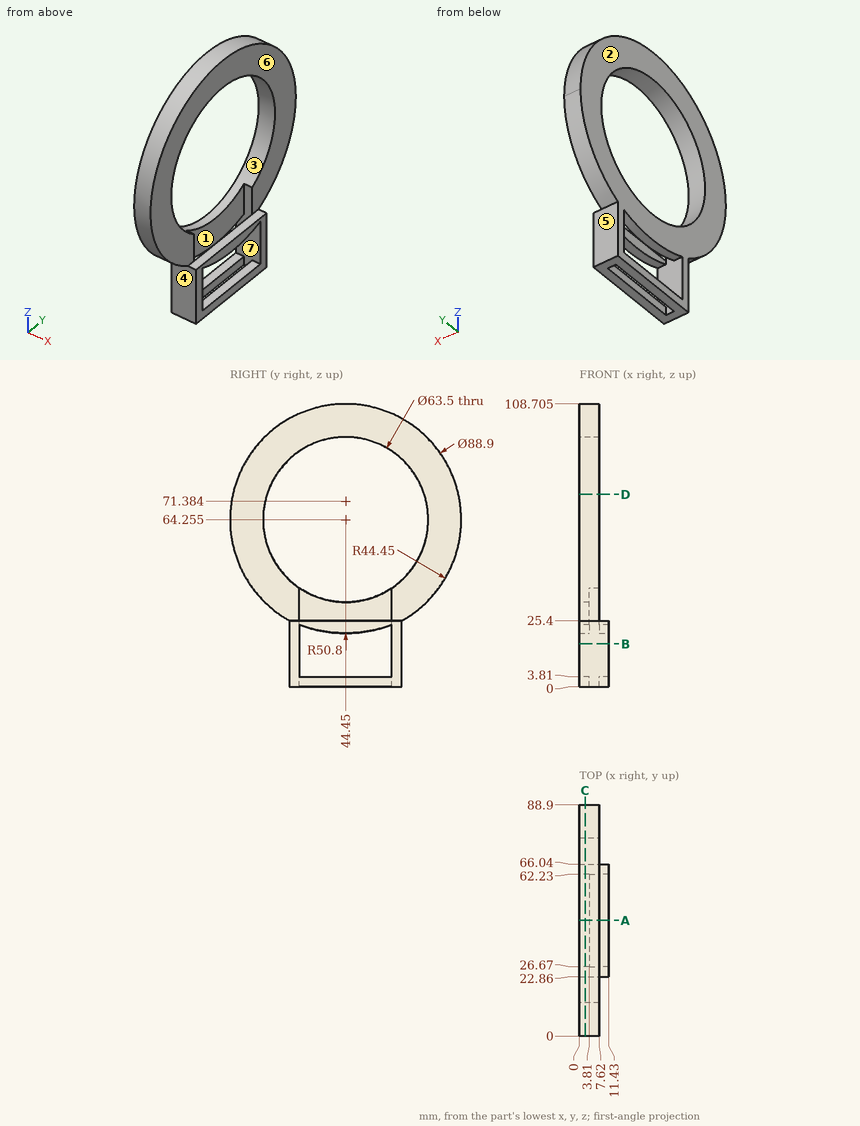
The figure shows three views and two pictorial views of one solid part (mm, origin at its lowest corner). Answer the questions. A direction names the side the tool comes from. Round coordinates to 2 decimals unless told otherwise and drop trailing zeros. Loops run counter-clockwise (first coordinate to the right, second up) from the corner with the lowest first, then second, coordinate; pieces in that order, holes last. Notation, with made-up numbers: M 20.5,53.25 L 52.5,53.25 A21 ccw 52.5,84.25 Z; hole C 8.5,-30 d5. An arc over 180 degrees is marked long. Use CSV: the item, a comma, the result in double quotes.
Q1. Section C-C, the plane x = 2.25 is taken. State how many separate pieces and enclosed holes the cut face has, then the cut area to 3 significant figures.
Determined:
separate pieces,"1"
enclosed holes,"2"
area,"3,340 mm2"
Q2. Section D-D, the plane z = 74 is taken. Determine the outline of the cut face in (x, y).
Determined:
outline,"M 0,1.08 L 7.62,1.08 L 7.62,14.23 L 0,14.23 Z; M 0,74.67 L 7.62,74.67 L 7.62,87.82 L 0,87.82 Z"
Q3. The mould has two halves that part along Z. Classify the marked faces 6 and 7: pulls with the +Z half, pulls with the -Z half, needs draft (parallel to the pull), parting line crosses it, or undercut.
Determined:
face 6,"needs draft"
face 7,"undercut"
Q4. Each of these flat-tipped pins is pushed along its axis until it touches: pin 1 (4 mm diameter, centred on x = 4, z = 63.5, fed in from +Y); pin 2 (3.5 mm diameter, centred on x = 7, z = 18, fed in from +Y); pin 3 (4 mm diameter, centred on x = 8.5, y = 45.5, fed in from +Z) (1 decimal); pin 4 (2 mm diameter, centred on x = 1.5, z = 38.5, fed in from +Y). Where does it stop, or does it pass through?
Determined:
pin 1,"y = 88.9"
pin 2,"y = 66.04"
pin 3,"z = 108.7"
pin 4,"y = 81.37"
Q5. Section A-A, the plane y = 44.45 is taken. Determine the outline of the cut face in (x, z) (1 decimal).
Determined:
outline,"M 0,0 L 3.8,0 L 3.8,3.8 L 0,3.8 Z; M 0,20.6 L 3.8,20.6 L 3.8,32.5 L 0,32.5 Z; M 0,96 L 7.6,96 L 7.6,108.7 L 0,108.7 Z; M 7.6,0 L 11.4,0 L 11.4,3.8 L 7.6,3.8 Z; M 7.6,20.6 L 11.4,20.6 L 11.4,25.4 L 7.6,25.4 Z"
Q6. A tool of negligible diameter and unlimited length cuts with its end or side. For the marked faces 1, 2, 3, 4 and 5, from which of +Z, -Z, +X, -X, +Y, -Y can it reach the whole face along a straight path? Write none if from no direction.
Determined:
face 1,"-Z"
face 2,"+Z, -Z, -X, +Y, -Y"
face 3,"+X, -X"
face 4,"-Z, +X, -X, -Y"
face 5,"-Z, +X, -X, +Y"
Q7. Consider L1, parallel to Y at x = 3, z = 14; L2, parallel to Z at x = 1, y = 58.5 (1 decimal); L3, parallel to Z at x = 3.75, y = 32 (1 decimal). Determine where each line is inside the solid, lowest interval first.
Determined:
L1,"22.86 to 26.67, 62.23 to 66.04"
L2,"0 to 3.8, 22.6 to 35.8, 92.7 to 106.4"
L3,"0 to 3.8, 22.1 to 35, 93.5 to 106.9"
Q8. Section B-B, the plane z = 16.5 is taken. Determine the outline of the cut face in (x, y).
Determined:
outline,"M 0,22.86 L 11.43,22.86 L 11.43,26.67 L 0,26.67 Z; M 0,62.23 L 11.43,62.23 L 11.43,66.04 L 0,66.04 Z"
